Geometry check sheet. Reference: the model listing, model coordinates, mm. Round coordinates to 2 decimals unless told otherwise and drop trailing zeros. Order: outer loops, then holes, each group sorted by start corner. A loop starts at its lowest first (then second) coordinate and runs counter-clockwise, first axis right, second up. Notation, with made-up numbers: (-2, 18) - (55, 18) arc R24 ccw to (55, 28) - close; hole circle Ø7 at (63.5, 17). An arc over 180 degrees is marked (long way). One line per question, with ' | ' between items. Start each with the question number.
Q1. Sectioned sample at A-A, the plane x = 26. Enter the section's corners in (y, z).
Q2. Gauge pin test, flat ends, axial feed: P1, Ø3, axis at x = -26, z = -14.5, coming from the -Y side; P2, Ø15.5, axis at x = 17.526, z = 4.699, coming from the -Y side. Record the tip position at first contact, or that the pin passes through.
Q3. Sectioned sample at B-B, the plane z = 14.5. Enter the section's corners in (x, y), then the cut area to 3 significant figures.
Q4. Material ranges on line 1 along X through (y, z) = (0.7, 14.5); line 2 along X through (y, z) = (2.6, -14); line 3 along Z through (x, y) = (19, 1.3), recorded low to high.
Q5. Sectioned sample at C-C, the plane y = 0.55. Enter the section's corners in (x, z), then the cut area to 3 significant figures.
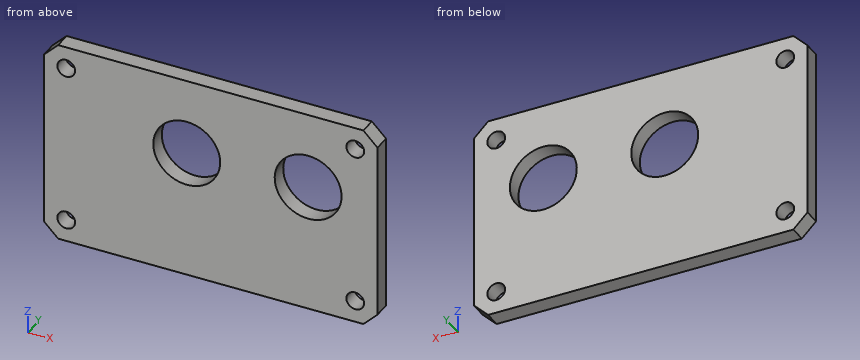
```python
from build123d import *

# Parameters (mm, degrees)
SKETCH1_W           = 60
SKETCH1_H           = 37
BOSS_EXTRUDE1_DEPTH = 2.9972
SKETCH2_R           = 1.6
CUT_EXTRUDE1_DEPTH  = 36.372774952
SKETCH3_R           = 6.0198
CUT_EXTRUDE2_DEPTH  = 36.372774952
CHAMFER1_SIZE       = 2.54


with BuildPart() as part:
    # Sketch1 → Boss-Extrude1 (new body)
    with BuildSketch(Plane(origin=(0, 0, 0), x_dir=(1, 0, 0), z_dir=(0, 1, 0))):
        Rectangle(SKETCH1_W, SKETCH1_H)
    extrude(amount=BOSS_EXTRUDE1_DEPTH)

    # Sketch2 → Cut-Extrude1 (cut, through all)
    with BuildSketch(Plane(origin=(0, 2.9972, 0), x_dir=(1, 0, 0), z_dir=(0, 1, 0))):
        with Locations(Location((-26, 14.5, 0), (0, 0, 270))):
            Circle(SKETCH2_R)
        with Locations(Location((-26, -14.5, 0), (0, 0, 270))):
            Circle(SKETCH2_R)
        with Locations(Location((26, -14.5, 0), (0, 0, 270))):
            Circle(SKETCH2_R)
        with Locations(Location((26, 14.5, 0), (0, 0, 270))):
            Circle(SKETCH2_R)
    extrude(amount=-CUT_EXTRUDE1_DEPTH, mode=Mode.SUBTRACT)

    # Sketch3 → Cut-Extrude2 (cut, through all)
    with BuildSketch(Plane(origin=(0, 2.9972, 0), x_dir=(1, 0, 0), z_dir=(0, 1, 0))):
        with Locations(Location((-4.318, -4.699, 0), (0, 0, 270))):
            Circle(SKETCH3_R)
        with Locations(Location((17.526, -4.699, 0), (0, 0, 270))):
            Circle(SKETCH3_R)
    extrude(amount=-CUT_EXTRUDE2_DEPTH, mode=Mode.SUBTRACT)

    # Chamfer1
    chamfer1_edges = [part.edges().sort_by_distance(p)[0] for p in [
        (30, 1.4986, 18.5),
        (-30, 1.4986, 18.5),
        (-30, 1.4986, -18.5),
        (30, 1.4986, -18.5),
    ]]
    chamfer(chamfer1_edges, length=CHAMFER1_SIZE)


solid = part.part
```
Determined:
1) outline: (0, -18.5) - (3, -18.5) - (3, -16.1) - (0, -16.1) - close; (0, -12.9) - (3, -12.9) - (3, 12.9) - (0, 12.9) - close; (0, 16.1) - (3, 16.1) - (3, 18.5) - (0, 18.5) - close
2) P1: passes through | P2: stops at y = 0
3) outline: (-30, 0) - (-27.6, 0) - (-27.6, 3) - (-30, 3) - close; (-24.4, 0) - (24.4, 0) - (24.4, 3) - (-24.4, 3) - close; (27.6, 0) - (30, 0) - (30, 3) - (27.6, 3) - close | area: 161 mm2
4) line 1: x = -30 to -27.6, -24.4 to 24.4, 27.6 to 30 | line 2: x = -30 to -27.52, -24.48 to 24.48, 27.52 to 30 | line 3: z = -18.5 to -1.14, 10.54 to 18.5
5) outline: (-30, -15.96) - (-27.46, -18.5) - (27.46, -18.5) - (30, -15.96) - (30, 15.96) - (27.46, 18.5) - (-27.46, 18.5) - (-30, 15.96) - close; hole circle Ø3.2 at (-26, -14.5); hole circle Ø3.2 at (-26, 14.5); hole circle Ø12.04 at (-4.32, 4.7); hole circle Ø12.04 at (17.53, 4.7); hole circle Ø3.2 at (26, -14.5); hole circle Ø3.2 at (26, 14.5) | area: 1,950 mm2
